The model under review builds one solid part; all positions refer to its coordinate system, in mm. Face numbers are marked on the shaded views. Round coordinates to 2 decimals unless told otherwise and drop trailing zeros. Write each loop counter-clockwise with the first axis right and the second up, starting at its lowest first coordinate (ties: lowest second). Pieces come first, ordered by that corner, then holes. Notation, with made-up numbers: (55.25, 78.25) - (88.25, 78.25) arc R23 cw to (88.25, 113.25) - close; hole circle Ø1 at (24, 21). An arc over 180 degrees is marked (long way). Write each question's results on one line, items separated by ' | '.
```python
from build123d import *

# Parameters (mm, degrees)
F_3_0_213_DIAMETER_HOLE1_REACH  = 150.785
F_3_0_213_DIAMETER_HOLE1_BORE_R = 2.7051
CIRPATTERN1_COUNT               = 8


with BuildPart() as part:
    # Sketch1 → Revolve2 (revolve)
    with BuildSketch(Plane.XY, mode=Mode.PRIVATE) as revolve2_sk:
        with BuildLine():
            Line((-63.5, 0), (-63.5, 50.8))
            Line((-63.5, 50.8), (-60.325, 50.8))
            Line((-60.325, 50.8), (-60.325, 38.1))
            ThreePointArc((-60.325, 38.1), (-33.051376431, 48.308044626), (-4.2164, 52.382213484))
            Line((-4.2164, 52.382213484), (-4.2164, 45.393561735))
            ThreePointArc((-4.2164, 45.393561735), (-24.682494429, 43.041960117), (-44.499135715, 37.412414884))
            ThreePointArc((-44.499135715, 37.412414884), (-53.477680006, 30.42702697), (-56.874265357, 19.570088643))
            Line((-56.874265357, 19.570088643), (-60.325, 0))
            Line((-60.325, 0), (-63.5, 0))
        make_face()
    revolve(revolve2_sk.sketch.rotate(Axis((0, 127.060987048, 0), (0, -1, 0)), 270), axis=Axis((0, 127.060987048, 0), (0, -1, 0)))

    # #3 (0.213) Diameter Hole1 bore (on position points) → #3 (0.213) Diameter Hole1 (cut, up to next)
    with BuildSketch(Plane(origin=(0, 44.45, 63.5), x_dir=(1, 0, 0), z_dir=(0, 0, 1)), mode=Mode.PRIVATE) as f_3_0_213_diameter_hole1_sk1:
        Circle(F_3_0_213_DIAMETER_HOLE1_BORE_R)
    f_3_0_213_diameter_hole1_tool1 = extrude(f_3_0_213_diameter_hole1_sk1.sketch, amount=-F_3_0_213_DIAMETER_HOLE1_REACH, mode=Mode.PRIVATE) & part.part
    f_3_0_213_diameter_hole1 = f_3_0_213_diameter_hole1_tool1.solids().sort_by_distance((0, 44.45, 63.5))[0]
    add(f_3_0_213_diameter_hole1, mode=Mode.SUBTRACT)

    # CirPattern1: #3 (0.213) Diameter Hole1 ×8 about axis
    cirpattern1_axis = Axis((0, 127.060987048, 0), (0, -1, 0))
    for i in range(1, CIRPATTERN1_COUNT):
        add(f_3_0_213_diameter_hole1.rotate(cirpattern1_axis, i * 360 / CIRPATTERN1_COUNT), mode=Mode.SUBTRACT)


solid = part.part
```
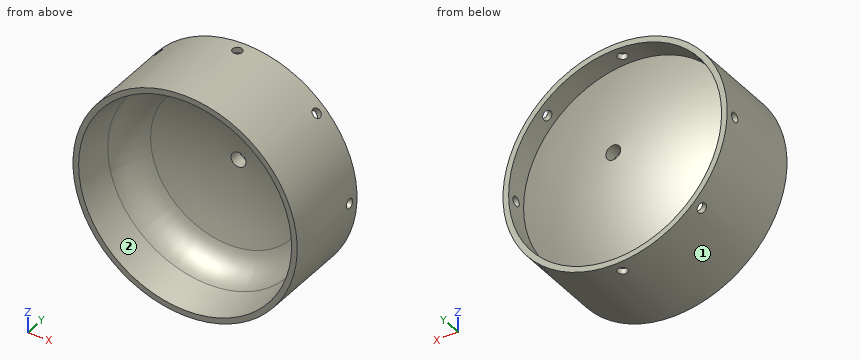
Q1. We need section A-A (x = 0). State the section outline as (y, z) points (3 decimals).
Evaluation:
outline: (0, -63.5) - (41.745, -63.5) - (41.745, -60.325) - (38.1, -60.325) arc R133.985 ccw to (52.382, -4.216) - (45.394, -4.216) arc R127 cw to (37.412, -44.499) arc R19.05 cw to (19.57, -56.874) - (0, -60.325) - close; (0, 60.325) - (19.57, 56.874) arc R19.05 cw to (37.412, 44.499) arc R127 cw to (45.394, 4.216) - (52.382, 4.216) arc R133.985 ccw to (38.1, 60.325) - (41.745, 60.325) - (41.745, 63.5) - (0, 63.5) - close; (47.155, -63.5) - (50.8, -63.5) - (50.8, -60.325) - (47.155, -60.325) - close; (47.155, 60.325) - (50.8, 60.325) - (50.8, 63.5) - (47.155, 63.5) - close
Q2. The part is to be moulded in two halves that separate along Z. For the marked faces 1 and 2, say which applies: released by +Z, released by -Z, zero draft, split by the parting line, or undercut.
Evaluation:
face 1: split by the parting line | face 2: undercut
Q3. We need section B-B (z = 0). State the section outline as (x, y) points (3 decimals), plus the area to 3 significant figures.
Evaluation:
outline: (-63.5, 0) - (-60.325, 0) - (-56.874, 19.57) arc R19.05 cw to (-44.499, 37.412) arc R127 cw to (-4.216, 45.394) - (-4.216, 52.382) arc R133.985 ccw to (-60.325, 38.1) - (-60.325, 41.745) - (-63.5, 41.745) - close; (-63.5, 47.155) - (-60.325, 47.155) - (-60.325, 50.8) - (-63.5, 50.8) - close; (4.216, 45.394) arc R127 cw to (44.499, 37.412) arc R19.05 cw to (56.874, 19.57) - (60.325, 0) - (63.5, 0) - (63.5, 41.745) - (60.325, 41.745) - (60.325, 38.1) arc R133.985 ccw to (4.216, 52.382) - close; (60.325, 47.155) - (63.5, 47.155) - (63.5, 50.8) - (60.325, 50.8) - close | area: 1,310 mm^2
Q4. Insertion check: P1, Ø6, axis at x = 7.5, y = 14.5, coming from the -Z side; P2, Ø5, axis at x = 0, z = 0, coming from the -Y side; P3, Ø6, axis at x = 25, z = 45.5, coming from the -Y side; P4, Ø4, axis at x = 16, z = -3.5, coming from the -Y side. Each pin has a flat end and moves straight along its axis. Give the tip position at first contact, or say it passes through.
Evaluation:
P1: stops at z = -63.34 | P2: passes through | P3: stops at y = 27.98 | P4: stops at y = 44.13
Q5. We need section C-C (y = 32). State the section outline as (x, z) points, plus the area to 3 significant figures.
Evaluation:
outline: circle Ø127 at (0, 0); hole circle Ø104.52 at (0, 0) | area: 4,090 mm^2
Q6. For probe 1 along Y at (x, z) = (-62, 0); probe 2 along Z at (x, y) = (-19, 5); probe 3 along Z at (x, y) = (-19, 17.5), list the stretches that pass through material, from the lowest coordinate up.
Evaluation:
probe 1: y = 0 to 41.74, 47.16 to 50.8 | probe 2: z = -60.59 to -56.33, 56.33 to 60.59 | probe 3: z = -60.59 to -53.99, 53.99 to 60.59
Q7. We need section D-D (y = 3). State the section outline as (x, z) points, plus the area to 3 significant figures.
Evaluation:
outline: circle Ø127 at (0, 0); hole circle Ø119.59 at (0, 0) | area: 1,430 mm^2
